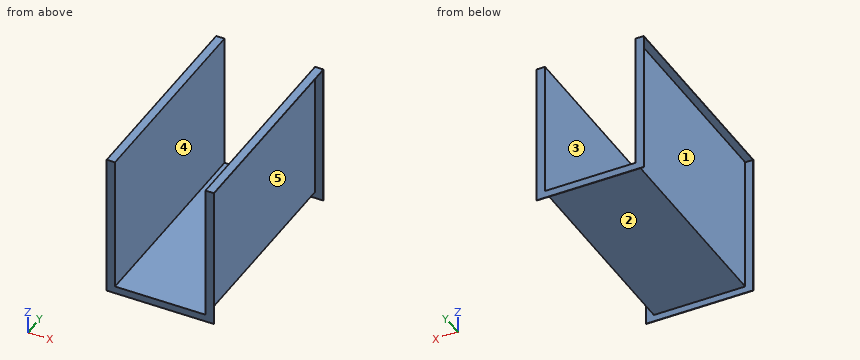
from build123d import *

# Parameters (mm, degrees)
F1_DEPTH = 1500
F2_T     = -3
F3_W     = 60
F3_H     = 1500
F4_DEPTH = 3
F6_DEPTH = 3
F8_DEPTH = 3


with BuildPart() as f1:
    # F0 (on Front) → F1 (new body)
    with BuildSketch(Plane.XZ):
        Polygon((330, 990), (-330, 990), (-330, 0), (0, 0), (330, 0), align=None)
    extrude(amount=F1_DEPTH)

    # F2
    f2_openings = [f1.faces().sort_by_distance(p)[0] for p in [
        (0, -1500, 495),
        (0, -750, 990),
        (0, 0, 495),
    ]]
    offset(amount=F2_T, openings=f2_openings)

    # F3 (on face) → F4 (join)
    with BuildSketch(Plane.XY.offset(990)):
        with Locations((-357, -750)):
            Rectangle(F3_W, F3_H)
        with Locations((357, -750)):
            Rectangle(F3_W, F3_H)
    extrude(amount=-F4_DEPTH)

    # F5 (on face) → F6 (join)
    with BuildSketch(Plane(origin=(0, 0, 0), x_dir=(-1, 0, 0), z_dir=(0, 1, 0))):
        Polygon((387, 990), (327, 990), (327, 3), (-327, 3), (-327, 990), (-387, 990), (-387, -50), (-75.369177, -50), (387, -50), align=None)
    extrude(amount=F6_DEPTH)

    # F7 (on face) → F8 (join)
    with BuildSketch(Plane.XZ.offset(1500)):
        Polygon((387, -50), (387, 990), (327, 990), (327, 3), (-327, 3), (-327, 990), (-387, 990), (-387, -50), (-70.356654, -50), align=None)
    extrude(amount=F8_DEPTH)


solid = f1.part
The model under review builds one solid part; all positions refer to its coordinate system, in mm. Face numbers are marked on the shaded views. A direction names the side the tool comes from. Round coordinates to 2 decimals unless told otherwise and drop trailing zeros. Loops run counter-clockwise (first coordinate to the right, second up) from the corner with the lowest first, then second, coordinate; pieces in that order, holes last. Notation, with made-up numbers: (28, -2) - (32, -2) arc R18 ccw to (32, 6) - close; hole circle Ø5 at (-25, -26). An arc over 180 degrees is marked (long way). Use CSV: the item, a comma, the result in double quotes.
(1) Take a section at A-A, the plane z = 569. Give the boundary of the cut face in (x, y).
Working result:
outline,"(-387, -1503) - (-327, -1503) - (-327, 3) - (-387, 3) - (-387, 0) - (-330, 0) - (-330, -1500) - (-387, -1500) - close; (327, -1503) - (387, -1503) - (387, -1500) - (330, -1500) - (330, 0) - (387, 0) - (387, 3) - (327, 3) - close"
(2) The part is to be moulded in two halves that separate along Y. For the marked faces 4 and 5, say which applies: pulls with the +Y half, pulls with the -Y half, needs draft (parallel to the pull), parting line crosses it, or undercut.
Working result:
face 4,"needs draft"
face 5,"undercut"
(3) Machinability: for the marked faces 1, 2 and 3, which of the approach directions +Z, -Z, +X, -X, +Y, -Y give a long, thin tool a straight path to every point of the face, cutting with its end or side? Answer none if there is none.
Working result:
face 1,"-Z, -X"
face 2,"-Z, +X, -X"
face 3,"+Z, +Y, -Y"
(4) For line 1 (X direction, y = -1276, z = 567.5); line 2 (Y direction, x = 338, z = 444.5); line 3 (Z direction, x = -144.5, y = -439.5), list the stretches that pass through material, from the lowest coordinate up.
Working result:
line 1,"x = -330 to -327, 327 to 330"
line 2,"y = -1503 to -1500, 0 to 3"
line 3,"z = 0 to 3"
(5) Clearance check with flat-ended pins moving along their axes: P1, Ø12, axis at x = -218.5, y = -649, coming from the +Z side; P2, Ø2, axis at y = -244.5, z = 823, coming from the -X side; P3, Ø12, axis at y = -1320, z = 457.5, coming from the +X side. State where each tip first meets the part, or that it passes through.
Working result:
P1,"stops at z = 3"
P2,"stops at x = -330"
P3,"stops at x = 330"
(6) Take a section at C-C, the plane x = -211.5. Give the boundary of the cut face in (y, z), plus the area to 3 significant figures.
Working result:
outline,"(-1503, -50) - (-1500, -50) - (-1500, 0) - (0, 0) - (0, -50) - (3, -50) - (3, 3) - (-1503, 3) - close"
area,"4,820 mm^2"
(7) Take a section at B-B, the plane y = -1380. Give the boundary of the cut face in (x, z).
Working result:
outline,"(-387, 987) - (-330, 987) - (-330, 0) - (330, 0) - (330, 987) - (387, 987) - (387, 990) - (327, 990) - (327, 3) - (-327, 3) - (-327, 990) - (-387, 990) - close"
